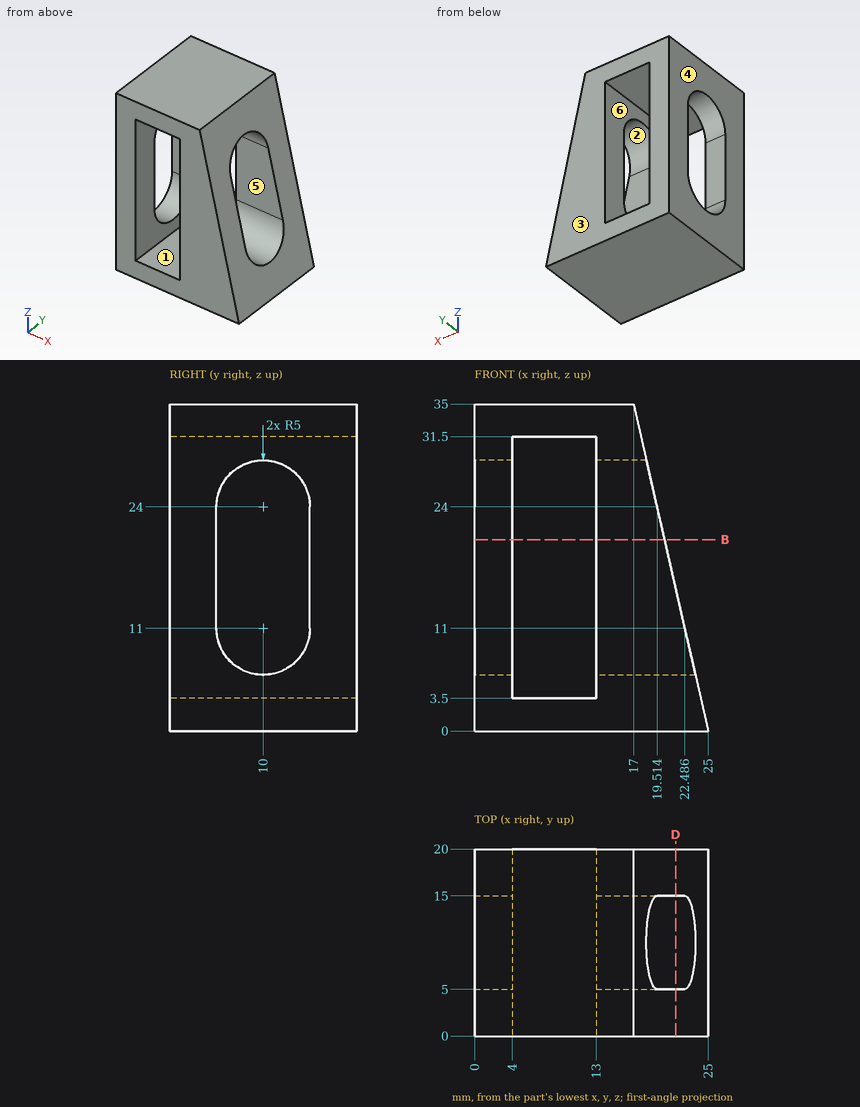
The figure shows three views and two pictorial views of one solid part (mm, origin at its lowest corner). Answer the questions. A direction names the side the tool comes from. Give positions to 0.01 mm unless a question says otherwise; leave off trailing zeros. Order: outer loops, then holes, each group sorted by start corner. A loop starts at its lowest first (then second) coordinate and runs counter-clockwise, first axis right, second up. Notation, with made-up numbers: M 45,-1 L 69,-1 A26 ccw 69,19 Z; hole C -29,-23.75 d6. An arc over 180 degrees is marked long. Return JSON: item names as keys, results as strings.
Q1. Find section B-B, the plane z = 20.5. Write down the section's boundary in (x, y), and give its area (3 significant figures).
Answer below:
{"outline": "M 0,0 L 4,0 L 4,5 L 0,5 Z; M 0,15 L 4,15 L 4,20 L 0,20 Z; M 13,0 L 20.31,0 L 20.31,5 L 13,5 Z; M 13,15 L 20.31,15 L 20.31,20 L 13,20 Z", "area": "113 mm^2"}
Q2. The mould has two halves that part along Y. Classify the marked faces 1, 2 and 3: pulls with the +Y half, pulls with the -Y half, needs draft (parallel to the pull), parting line crosses it, or undercut.
Answer below:
{"face 1": "needs draft", "face 2": "undercut", "face 3": "pulls with the +Y half"}
Q3. Which of the six approach directions +Z, -Z, +X, -X, +Y, -Y give full straight-line access (tool end or side, diameter ignored) to the marked faces 4, 5 and 6?
Answer below:
{"face 4": "+Z, -Z, -X, +Y, -Y", "face 5": "+X, -X", "face 6": "+Y, -Y"}
Q4. Each of these flat-tipped pins is pushed along its axis until it touches: pin 1 (6 mm diameter, centred on x = 11, z = 13, fed in from +Y); pin 2 (10 mm diameter, centred on y = 8, z = 28, fed in from +X). Where does it stop, or does it pass through?
Answer below:
{"pin 1": "stops at y = 20", "pin 2": "stops at x = 19.51"}
Q5. Find the intervals of material crossed by line 1 along Z through (x, y) = (12, 4.5); line 2 along Y through (x, z) = (19.5, 22.5); line 3 along X through (y, z) = (3.75, 18) (1 decimal), in increasing order. Write a range as [from, to].
Answer below:
{"line 1": "z = [0, 3.5], [31.5, 35]", "line 2": "y = [0, 5], [15, 20]", "line 3": "x = [0, 4], [13, 20.9]"}
Q6. Find section D-D, the plane x = 21.5. Write down the section's boundary in (y, z), and give its area (3 significant figures).
Answer below:
{"outline": "M 0,0 L 20,0 L 20,15.31 L 15,15.31 L 15,11 A5 cw 5,11 L 5,15.31 L 0,15.31 Z", "area": "224 mm^2"}
